The listing builds one solid part. Answer for the finished solid, in the listing's coordinates (mm). Give positions to 0.01 mm unless a question says otherwise; leave off trailing zeros. Order: outer loops, then holes, each group sorted by start corner. A loop starts at its lowest first (then second) coordinate and runs counter-clockwise, first axis right, second up. Notation, with made-up numbers: (80.25, 40) -> (119.25, 40) arc R15 cw to (119.25, 59) -> close; hole circle Ø7 at (30, 40.5). An arc over 180 degrees is marked (long way). Write item = value, one per line. Start each with the question number.
```python
from build123d import *

# Parameters (mm, degrees)
F0_W     = 19.05
F0_H     = 6.35
F0_R     = 1.35255
F1_DEPTH = 6.35
F2_R     = 1.35255
F3_DEPTH = 6.35


with BuildPart() as f1:
    # F0 (on Top) → F1 (new body)
    with BuildSketch(Plane.XY):
        Rectangle(F0_W, F0_H)
        Circle(F0_R, mode=Mode.SUBTRACT)
    extrude(amount=F1_DEPTH)

    # F2 (on face) → F3 (cut, through all)
    with BuildSketch(Plane.XZ.offset(3.175)):
        with Locations((-6.35, 3.175)):
            Circle(F2_R)
        with Locations((6.35, 3.175)):
            Circle(F2_R)
    extrude(amount=-F3_DEPTH, mode=Mode.SUBTRACT)


solid = f1.part
```
Item 1: Consider L1, parallel to Z at x = -6.35, y = 0.75; L2, parallel to X at y = 2.5, z = 3.5 (3 decimals); L3, parallel to Y at x = 0, z = 4.25 (3 decimals). Determine where each line is inside the solid, lowest interval first. Write a range as from..to.
Item 2: A cutting plane is placed at D-D, the plane y = 1.75. Write down the section's boundary in (x, z) (3 decimals), plus the area to 3 significant figures.
Item 3: A cutting plane is placed at C-C, the plane z = 2. Write down the section's boundary in (x, y) (3 decimals).
Item 4: The mould has two halves that part along Y. Classify faces 1 (the cylindrical face through (1.29, 0.41, 3.13)), 2 (the flat face through (0, -3.175, 3)), 3 (the flat face through (-0.1, 1.5, 6.35)): +Y half, -Y half, draft (parallel to the pull), parting line (faces both ways), or undercut.
Item 5: A cutting plane is placed at B-B, the plane x = 0. Write down the section's boundary in (y, z) (3 decimals).
Item 6: A cutting plane is placed at A-A, the plane y = 0. Write down the section's boundary in (x, z) (3 decimals).
Check values:
q1.L1 = 0..1.82, 4.53..6.35
q1.L2 = -9.525..-7.663, -5.037..5.037, 7.663..9.525
q1.L3 = -3.175..-1.353, 1.353..3.175
q2.outline = (-9.525, 0) -> (9.525, 0) -> (9.525, 6.35) -> (-9.525, 6.35) -> close; hole circle Ø2.705 at (-6.35, 3.175); hole circle Ø2.705 at (6.35, 3.175)
q2.area = 109 mm^2
q3.outline = (-9.525, -3.175) -> (-7.02, -3.175) -> (-7.02, 3.175) -> (-9.525, 3.175) -> close; (-5.68, -3.175) -> (5.68, -3.175) -> (5.68, 3.175) -> (-5.68, 3.175) -> close; (7.02, -3.175) -> (9.525, -3.175) -> (9.525, 3.175) -> (7.02, 3.175) -> close; hole circle Ø2.705 at (0, 0)
q4.face_1 = undercut
q4.face_2 = -Y half
q4.face_3 = draft
q5.outline = (-3.175, 0) -> (-1.353, 0) -> (-1.353, 6.35) -> (-3.175, 6.35) -> close; (1.353, 0) -> (3.175, 0) -> (3.175, 6.35) -> (1.353, 6.35) -> close
q6.outline = (-9.525, 0) -> (-1.353, 0) -> (-1.353, 6.35) -> (-9.525, 6.35) -> close; (1.353, 0) -> (9.525, 0) -> (9.525, 6.35) -> (1.353, 6.35) -> close; hole circle Ø2.705 at (-6.35, 3.175); hole circle Ø2.705 at (6.35, 3.175)
